Here's how the part is built. I have some questions about the finished solid (model axes, mm). A direction names the side the tool comes from. Coordinates: 2 decimals unless noted, no trailing zeros. Loops run counter-clockwise (first coordinate to the right, second up) from the corner with the lowest first, then second, coordinate; pieces in that order, holes last. Notation, with made-up numbers: M 86,67 L 97,67 A13 ccw 97,77 Z; hole C 16.25,52.5 d10. An arc over 180 degrees is marked long. Use one line per item in the form item = value. Start each with the question number.
(1) Thinking about a two-plate mould opening in Z: for faces 1 (the flat face through (0, -32, 171)), 2 (the flat face through (126, -35, 79)), 3 (the flat face through (6, -55, 130)), which applies, +Z half, -Z half, draft (parallel to the pull), parting line (faces both ways), or undercut?
(2) Imagine slicing it at C-C, the plane y = -17.5. Please give me the cut outline in (x, z), and give its area (3 significant figures).
(3) Please list where these lines run through material, in increasing order: L1, parallel to X at y = -45, z = 15; L2, parallel to Z at x = 46, y = -23.5; L3, parallel to Z at x = 111.5, y = -59.5.
(4) On a 3-axis mill with a long thin cutter (end or side, diameter ignored), from which of +Z, -Z, +X, -X, +Y, -Y can I reach the whole of each face in a straight line? I mean faces 4 (the flat face through (11, -55, 15)), 5 (the flat face through (6, -35, 135)), 6 (the flat face through (46, -10, 9)). Say none if no direction works.
(5) Imagine slicing it at A-A, the plane y = -65. Please give me the cut outline in (x, z), and give its area (3 significant figures).
(6) Will these pins go through, and if not, where does the flat tip stop? P1, Ø5, axis at x = 106.5, y = -1.5, coming from the -Z side; P2, Ø9.5, axis at x = 94.5, z = 11, coming from the +Y side; P3, Ø6, axis at y = -7.5, z = 128, coming from the -X side; P4, Ø4, axis at x = 70, z = 150, coming from the +Y side.
(7) Imagine slicing it at D-D, the plane z = 151. Please give me the cut outline in (x, y).
(8) Imagine slicing it at B-B, the plane x = 116. Please give me the cut outline in (y, z).
Autodesk Inventor part; units mm, degrees
ref_plane "YZ Plane" through (0, 0, 0) normal (1, 0, 0) x (0, 1, 0)
ref_plane "XZ Plane" through (0, 0, 0) normal (0, 1, 0) x (-1, 0, 0)
ref_plane "XY Plane" through (0, 0, 0) normal (0, 0, 1) x (1, 0, 0)
sketch "Sketch1" plane through (0, 0, 0) normal (0, 1, 0) x (-1, 0, 0)
  point P0 (0, 0)
sketch "Sketch2" plane through (0, 0, 0) normal (0, 1, 0) x (-1, 0, 0)
  line L0 (0, 0) -> (-160, 0)
  line L1 (-160, 0) -> (-160, 210)
  line L2 (-160, 210) -> (0, 210)
  line L3 (0, 210) -> (0, 0)
  dimension "d0" = 160
  dimension "d1" = 210
extrude "Extrusion1" add sketch "Sketch2" against normal blind 55
sketch "Sketch3" plane through (0, 0, 0) normal (-1, 0, 0) x (0, 0, 1)
  line L0 (0, 0) -> (0, -55)
  line L1 (0, 0) -> (9, 0)
  line L2 (9, 0) -> (9, -10)
  line L3 (9, -10) -> (0, -10)
  line L4 (0, -10) -> (0, 0)
  line L5 (0, 0) -> (210, 0)
  line L6 (9, -10) -> (131, -10)
  line L7 (131, -10) -> (131, 0)
  line L8 (131, 0) -> (9, 0)
  line L9 (9, 0) -> (9, -10)
  dimension "d4" = 9
  dimension "d5" = 10
  dimension "d6" = 122
extrude "Extrusion2" cut sketch "Sketch3" against normal blind 122 contours L5 L7 L6 L2
sketch "Sketch4" plane through (160, 0, 210) normal (1, 0, 0) x (0, 0, -1)
  line L0 (210, 0) -> (210, -55)
  line L1 (210, -55) -> (0, -55)
  line L2 (0, -55) -> (0, 0)
  line L3 (0, 0) -> (210, 0)
  line L4 (210, 0) -> (210, -55)
extrude "Extrusion3" cut sketch "Sketch4" against normal blind 29
sketch "Sketch5" plane through (0, -10, 131) normal (0, 1, 0) x (1, 0, 0)
  line L0 (122, 122) -> (122, 0)
  line L1 (0, 122) -> (122, 122)
  line L2 (122, 122) -> (122, 0)
  line L3 (122, 0) -> (0, 0)
  line L4 (0, 0) -> (0, 122)
  point P0 (0, 131)
extrude "Extrusion4" cut sketch "Sketch5" against normal blind 25
sketch "Sketch6" plane through (0, -35, 131) normal (0, 1, 0) x (1, 0, 0)
  line L0 (0, 122) -> (122, 122)
  line L1 (0, 122) -> (11, 122)
  line L2 (11, 122) -> (11, 111)
  line L3 (11, 111) -> (0, 111)
  line L4 (0, 111) -> (0, 122)
  line L5 (122, 122) -> (122, 0)
  line L6 (122, 122) -> (111, 122)
  line L7 (111, 122) -> (111, 111)
  line L8 (111, 111) -> (122, 111)
  line L9 (122, 111) -> (122, 122)
  line L10 (11, 111) -> (111, 111)
  line L11 (111, 111) -> (111, 11)
  line L12 (111, 11) -> (11, 11)
  line L13 (11, 11) -> (11, 111)
  point P0 (0, 131)
  dimension "d13" = 11
  dimension "d14" = 11
  dimension "d15" = 11
  dimension "d16" = 11
  dimension "d17" = 100
extrude "Extrusion5" cut sketch "Sketch6" against normal blind 20 contours L10 L11 L12 L13
sketch "Sketch7" plane through (0, -35, 131) normal (0, 1, 0) x (1, 0, 0)
  line L0 (11, 11) -> (11, 111)
  line L1 (0, 122) -> (122, 122)
  line L2 (11, 111) -> (111, 111)
  line L3 (111, 111) -> (111, 122)
  line L4 (111, 122) -> (11, 122)
  line L5 (11, 122) -> (11, 111)
  line L6 (0, 0) -> (0, 122)
  line L7 (11, 111) -> (0, 111)
  line L8 (0, 111) -> (0, 11)
  line L9 (0, 11) -> (11, 11)
  line L10 (11, 11) -> (11, 111)
  line L11 (111, 111) -> (111, 11)
  line L12 (122, 122) -> (122, 0)
  line L13 (111, 111) -> (122, 111)
  line L14 (122, 111) -> (122, 11)
  line L15 (122, 11) -> (111, 11)
  line L16 (111, 11) -> (111, 111)
  line L17 (111, 11) -> (11, 11)
  line L18 (11, 11) -> (111, 11)
  line L19 (111, 11) -> (111, 0)
  line L20 (111, 0) -> (11, 0)
  line L21 (11, 0) -> (11, 11)
  point P0 (0, 131)
  dimension "d20" = 100
  dimension "d21" = 100
  dimension "d22" = 100
  dimension "d23" = 11
extrude "Extrusion6" cut sketch "Sketch7" against normal blind 20 contours L9 L6 L7 L0 | L17 L19 L20 L21 | L5 L1 L3 L2 | L11 L13 L12 L15
sketch "Sketch8" plane through (0, 0, 0) normal (0, 1, 0) x (1, 0, 0)
  line L0 (0, 0) -> (131, 0)
  line L1 (0, -9) -> (122, -9)
  line L2 (131, 0) -> (111, 0)
  line L3 (111, 0) -> (111, -9)
  line L4 (111, -9) -> (131, -9)
  line L5 (131, -9) -> (131, 0)
  line L6 (111, 0) -> (11, 0)
  line L7 (11, 0) -> (11, -9)
  line L8 (11, -9) -> (111, -9)
  line L9 (111, -9) -> (111, 0)
  line L10 (131, -9) -> (122, -9)
  line L11 (122, -9) -> (122, -119)
  line L12 (122, -119) -> (131, -119)
  line L13 (131, -119) -> (131, -9)
  dimension "d26" = 20
  dimension "d27" = 100
  dimension "d28" = 9
  dimension "d29" = 110
extrude "Extrusion7" cut sketch "Sketch8" against normal blind 10 contours L0 L3 L1 L7 | L13 L12 L11 L4
sketch "Sketch10" plane through (0, -35, 9) normal (0, 0, 1) x (1, 0, 0)
  line L0 (111, 35) -> (131, 35)
  line L1 (131, 35) -> (122, 35)
  line L2 (122, 35) -> (122, 25)
  line L3 (122, 25) -> (131, 25)
  line L4 (131, 25) -> (131, 35)
  point P0 (0, 35)
extrude "Extrusion8" add sketch "Sketch10" along normal blind 11
sketch "Sketch11" plane through (122, 0, 131) normal (0, 0, -1) x (-1, 0, 0)
  line L0 (0, 0) -> (122, 0)
  line L1 (0, 0) -> (111, 0)
  line L2 (111, 0) -> (111, -10)
  line L3 (111, -10) -> (0, -10)
  line L4 (0, -10) -> (0, 0)
  dimension "d38" = 111
  dimension "d39" = 10
extrude "Extrusion9" cut sketch "Sketch11" against normal blind 80
sketch "Sketch12" plane through (0, -55, 210) normal (0, 0, 1) x (1, 0, 0)
  line L0 (122, 45) -> (11, 45)
  line L1 (11, 45) -> (11, 20)
  line L2 (131, 0) -> (0, 0)
  line L3 (11, 20) -> (111, 20)
  line L4 (111, 20) -> (111, 0)
  line L5 (111, 0) -> (11, 0)
  line L6 (11, 0) -> (11, 20)
  point P0 (0, 55)
  dimension "d42" = 25
  dimension "d43" = 100
extrude "Extrusion10" cut sketch "Sketch12" against normal blind 220
sketch "Sketch13" plane through (122, 0, 0) normal (-1, 0, 0) x (0, 0, 1)
  line L0 (0, -55) -> (210, -55)
  line L1 (20, -35) -> (120, -35)
  line L2 (120, -35) -> (120, -55)
  line L3 (120, -55) -> (20, -55)
  line L4 (20, -55) -> (20, -35)
  point P0 (0, 0)
  dimension "d46" = 100
extrude "Extrusion11" cut sketch "Sketch13" against normal blind 9
sketch "Sketch14" plane through (0, -35, 9) normal (0, 0, 1) x (1, 0, 0)
  line L0 (0, 35) -> (11, 35)
  line L1 (0, 35) -> (11, 35)
  line L2 (11, 35) -> (11, 0)
  line L3 (11, 0) -> (0, 0)
  line L4 (0, 0) -> (0, 35)
  line L5 (111, 25) -> (11, 25)
  line L6 (111, 0) -> (122, 0)
  line L7 (11, 25) -> (122, 25)
  line L8 (122, 25) -> (122, 0)
  line L9 (122, 0) -> (11, 0)
  line L10 (11, 0) -> (11, 25)
  line L11 (111, 25) -> (111, 35)
  line L12 (111, 35) -> (122, 35)
  line L13 (122, 35) -> (122, 25)
  line L14 (122, 25) -> (111, 25)
  line L15 (111, 25) -> (111, 35)
sketch "Sketch15" plane through (0, -35, 20) normal (0, 0, 1) x (1, 0, 0)
  line L0 (11, 0) -> (11, -20)
  line L1 (0, -20) -> (11, -20)
  line L2 (11, -20) -> (11, 0)
  line L3 (11, 0) -> (0, 0)
  line L4 (0, 0) -> (0, -20)
  line L5 (131, 0) -> (131, -20)
  line L6 (111.5686, -20) -> (131, -20)
  line L7 (131, -20) -> (131, 0)
  line L8 (131, 0) -> (111.5686, 0)
  line L9 (122, 35) -> (122, 25)
  line L10 (131, 25) -> (122, 25)
  line L11 (122, 35) -> (131, 35)
  line L12 (131, 35) -> (131, 25)
  line L13 (131, 25) -> (122, 25)
  line L14 (122, 25) -> (122, 35)
  line L15 (111, 0) -> (111, -20)
  line L16 (111, 0) -> (131, 0)
  line L17 (131, 0) -> (131, -20)
  line L18 (131, -20) -> (111, -20)
  line L19 (111, -20) -> (111, 0)
  point P0 (0, 35)
extrude "Extrusion12" add sketch "Sketch14" along normal blind 10
extrude "Extrusion13" add sketch "Sketch15" along normal blind 10
sketch "Sketch16" plane through (0, -35, 131) normal (0, 0, -1) x (-1, 0, 0)
  line L0 (-11, 35) -> (-11, 25)
  line L1 (-11, 0) -> (0, 0)
  line L2 (-11, 35) -> (0, 35)
  line L3 (0, 35) -> (0, 0)
  line L4 (0, 0) -> (-11, 0)
  line L5 (-11, 0) -> (-11, 35)
  line L6 (-11, 25) -> (-122, 25)
  line L7 (-122, 25) -> (-122, 0)
  line L8 (-11, 25) -> (-122, 25)
  line L9 (-122, 25) -> (-122, 0)
  line L10 (-122, 0) -> (-11, 0)
  line L11 (-11, 0) -> (-11, 25)
extrude "Extrusion14" cut sketch "Sketch16" against normal blind 10
sketch "Sketch18" plane through (131, -55, 120) normal (0, 0, -1) x (-1, 0, 0)
  line L0 (0, 0) -> (0, 20)
  line L1 (9, 20) -> (20, 20)
  line L2 (0, 0) -> (20, 0)
  line L3 (20, 0) -> (20, 20)
  line L4 (20, 20) -> (0, 20)
  line L5 (0, 20) -> (0, 0)
  line L6 (120, 20) -> (120, 0)
  line L7 (131, 20) -> (131, 0)
  line L8 (120, 0) -> (131, 0)
  line L9 (131, 0) -> (131, 20)
  line L10 (131, 20) -> (120, 20)
  line L11 (120, 20) -> (120, 0)
  point P0 (131, 55)
extrude "Extrusion15" cut sketch "Sketch18" against normal blind 10
sketch "Sketch19" plane through (131, 0, 119) normal (0, 0, -1) x (-1, 0, 0)
  line L0 (0, -10) -> (9, -10)
  line L1 (9, -10) -> (0, -10)
  line L2 (0, -10) -> (0, 0)
  line L3 (0, 0) -> (9, 0)
  line L4 (9, 0) -> (9, -10)
  point P0 (131, 0)
extrude "Extrusion16" cut sketch "Sketch19" against normal blind 11
sketch "Sketch20" plane through (0, -35, 19) normal (0, 0, 1) x (1, 0, 0)
  line L0 (11, 25) -> (111, 25)
  line L1 (111, 25) -> (92, 25)
  line L2 (92, 25) -> (92, 15)
  line L3 (92, 15) -> (111, 15)
  line L4 (111, 15) -> (111, 25)
  point P0 (0, 35)
  dimension "d59" = 19
  dimension "d60" = 10
extrude "Extrusion17" cut sketch "Sketch20" against normal blind 19
sketch "Sketch21" plane through (92, -20, 19) normal (1, 0, 0) x (0, 0, -1)
  line L0 (0, 0) -> (0, 10)
  line L1 (19, 10) -> (19, 0)
  line L2 (0, 0) -> (19, 0)
  line L3 (19, 0) -> (19, 10)
  line L4 (19, 10) -> (0, 10)
  line L5 (0, 10) -> (0, 0)
  point P0 (19, 20)
extrude "Extrusion18" cut sketch "Sketch21" against normal blind 10
sketch "Sketch22" plane through (0, -55, 0) normal (0, -1, 0) x (1, 0, 0)
  line L0 (11, 210) -> (0, 210)
  line L1 (11, 141) -> (11, 130)
  line L2 (0, 210) -> (11, 210)
  line L3 (11, 210) -> (11, 130)
  line L4 (11, 130) -> (0, 130)
  line L5 (0, 130) -> (0, 210)
  line L6 (11, 210) -> (111, 210)
  line L7 (131, 130) -> (131, 210)
  line L8 (111, 210) -> (131, 210)
  line L9 (131, 210) -> (131, 130)
  line L10 (131, 130) -> (111, 130)
  line L11 (111, 130) -> (111, 210)
  line L12 (0, 30) -> (0, 19)
  line L13 (11, 19) -> (11, 0)
  line L14 (0, 30) -> (11, 30)
  line L15 (11, 30) -> (11, 0)
  line L16 (11, 0) -> (0, 0)
  line L17 (0, 0) -> (0, 30)
  line L18 (131, 30) -> (131, 0)
  line L19 (111, 30) -> (131, 30)
  line L20 (131, 30) -> (131, 0)
  line L21 (131, 0) -> (111, 0)
  line L22 (111, 0) -> (111, 30)
extrude "Extrusion19" add sketch "Sketch22" along normal blind 20
sketch "Sketch23" plane through (0, 0, 0) normal (0, 1, 0) x (1, 0, 0)
  line L0 (0, 0) -> (11, 0)
  line L1 (11, -19) -> (11, 0)
  line L2 (0, 0) -> (11, 0)
  line L3 (11, 0) -> (11, -19)
  line L4 (11, -19) -> (0, -19)
  line L5 (0, -19) -> (0, 0)
  line L6 (111, 0) -> (111, -19)
  line L7 (122, -19) -> (122, -30)
  line L8 (111, 0) -> (122, 0)
  line L9 (122, 0) -> (122, -19)
  line L10 (122, -19) -> (111, -19)
  line L11 (111, -19) -> (111, 0)
  line L12 (131, -30) -> (131, 0)
  line L13 (122, -30) -> (131, -30)
  line L14 (131, -30) -> (131, 0)
  line L15 (131, 0) -> (122, 0)
  line L16 (122, 0) -> (122, -30)
  line L17 (122, -130) -> (122, -210)
  line L18 (131, -210) -> (131, -130)
  line L19 (122, -130) -> (131, -130)
  line L20 (131, -130) -> (131, -210)
  line L21 (131, -210) -> (122, -210)
  line L22 (122, -210) -> (122, -130)
  line L23 (11, -210) -> (11, -141)
  line L24 (0, -141) -> (11, -141)
  line L25 (11, -141) -> (11, -210)
  line L26 (11, -210) -> (0, -210)
  line L27 (0, -210) -> (0, -141)
extrude "Extrusion20" add sketch "Sketch23" along normal blind 10
properties part number "120mmLaptopStand-Right"
Answer:
q1.face_1 = draft
q1.face_2 = undercut
q1.face_3 = undercut
q2.outline = M 0,0 L 82,0 L 82,19 L 0,19 Z; M 0,141 L 122,141 L 122,19 L 111,19 L 111,0 L 131,0 L 131,210 L 0,210 Z
q2.area = 12,100 mm²
q3.L1 = 0 to 11, 111 to 131
q3.L2 = 0 to 19, 141 to 210
q3.L3 = 0 to 30, 130 to 210
q4.face_4 = +Z, -Z, -Y
q4.face_5 = -X, +Y
q4.face_6 = +Z, -Z, +Y
q5.outline = M 0,0 L 11,0 L 11,30 L 0,30 Z; M 0,130 L 11,130 L 11,210 L 0,210 Z; M 111,0 L 131,0 L 131,30 L 111,30 Z; M 111,130 L 131,130 L 131,210 L 111,210 Z
q5.area = 3,410 mm²
q6.P1 = through
q6.P2 = -20
q6.P3 = 122
q6.P4 = -10
q7.outline = M 0,-75 L 11,-75 L 11,-35 L 111,-35 L 111,-75 L 131,-75 L 131,10 L 122,10 L 122,-10 L 11,-10 L 11,10 L 0,10 Z
q8.outline = M -75,0 L 10,0 L 10,19 L -35,19 L -35,30 L -75,30 Z; M -75,130 L -35,130 L -35,141 L -10,141 L -10,210 L -75,210 Z
